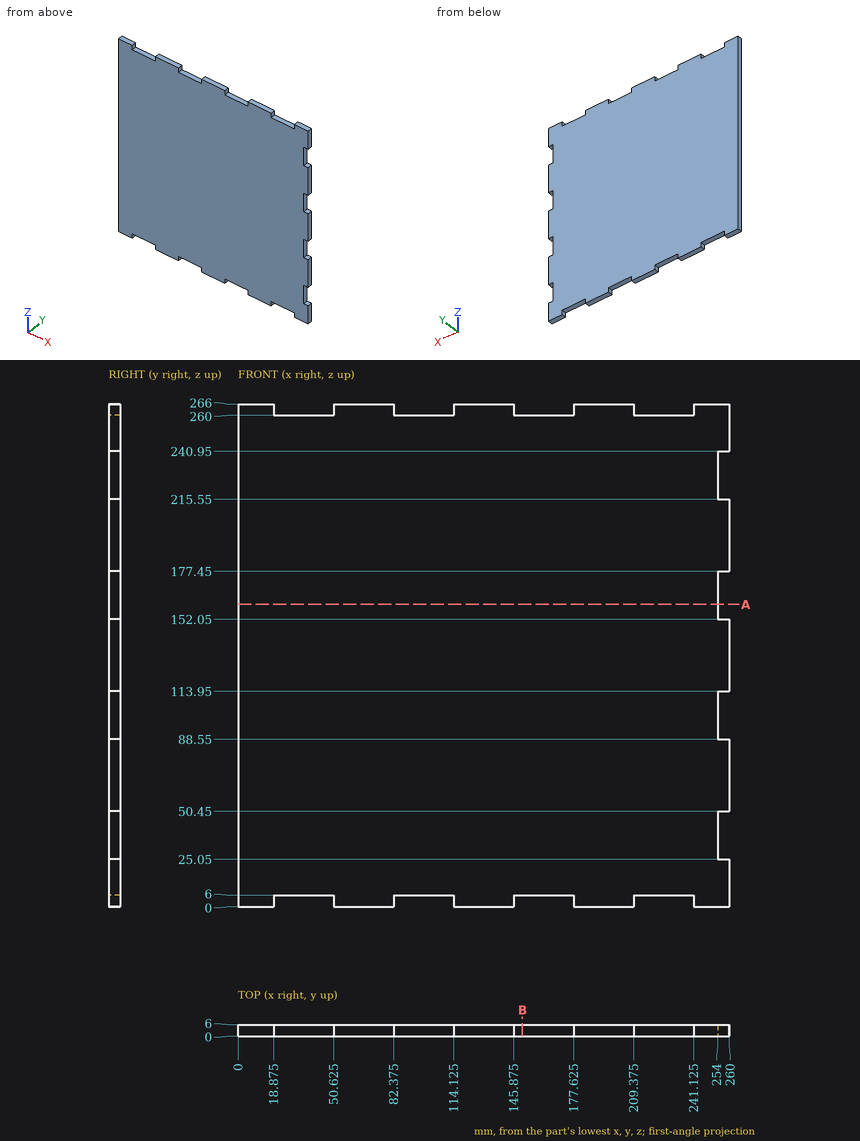
Source: three-view drawing plus pictorial views. Frame: mm from the lowest corner of the part. Round coordinates to 2 decimals unless told otherwise and drop trailing zeros. Loops run counter-clockwise (first coordinate to the right, second up) from the corner with the lowest first, then second, coordinate; pieces in that order, holes last.
Q1. Section A-A, the plane z = 160. Return loops of the section in (x, y), plus the area to 3 significant figures.
Q2. Section B-B, the plane x = 150.5. Return loops of the section in (y, z).
Q3. First-contact query: P1, Ø1.5, axis at x = 120, y = 1, coming from the -Z side; P2, Ø3, axis at x = 34.5, y = 1.5, coming from the -Z side; P3, Ø3, axis at x = 89, y = 5, coming from the +Z side; P4, Ø3, axis at y = 3, z = 107, coming from the +X side. Flat tips, straight axial feed; report the tip coordinate or a pass-through.
Q4. Ray query, line 1 (X direction, y = 1.25, z = 224.5); line 2 (Z direction, x = 43.5, y = 5.15). Return the intervals inside material, ascending.
Solutions:
1. outline: (0, 0) - (254, 0) - (254, 6) - (0, 6) - close
1. area: 1,520 mm2
2. outline: (0, 6) - (6, 6) - (6, 260) - (0, 260) - close
3. P1: stops at z = 0
3. P2: stops at z = 6
3. P3: stops at z = 260
3. P4: stops at x = 254
4. line 1: x = 0 to 254
4. line 2: z = 6 to 260
